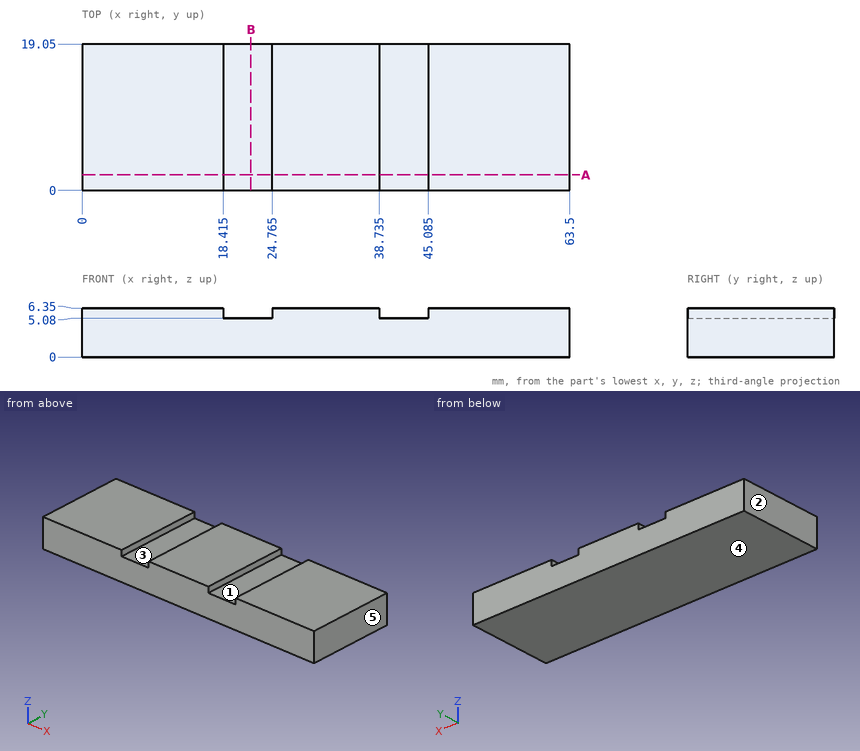
Job drawing, mm, ordinate dimensions from the low corner. One solid piece. A direction names the side the tool comes from. Coordinates: 2 decimals unless noted, no trailing zeros. Order: outer loops, then holes, each group sorted by start corner. A loop starts at its lowest first (then second) coordinate and runs counter-clockwise, first axis right, second up. Notation, with made-up numbers: (-28, -2.75) -> (27, -2.75) arc R28 ccw to (27, 21.25) -> close; hole circle Ø8 at (-27.5, 41.5). An arc over 180 degrees is marked (long way). Answer in a Markdown table with one row per item. Add a question column.
Q1. Wall check: line 1 along X through (y, z) = (8, 5.5) (3 decimals); line 2 along Z through (x, y) = (21, 1). Give the ranges that are in metal, low to high. Write a range as [from, to].
Q2. Band-saw the part on A-A, the plane y = 2. List the corners of the cut face in (x, z) (3 decimals).
Q3. Drop a flat-ended pin along its axis: pin 1 (1.9 mm diameter, centred on x = 23, y = 8.5, fed in from +Z). Give the stop position or say it passes through.
Q4. Band-saw the part on B-B, the plane x = 22. List the corners of the cut face in (y, z).
Q5. Mould opens along X. For the marked faces 3, 4 and 5 say: +X half, -X half, draft (parallel to the pull), parting line (faces both ways), or undercut.
Q6. Which spindle directions (+Z, -Z, +X, -X, +Y, -Y) get a long thin tool onto all of the face, cutting with end or side? Do the marked faces 1 and 2. Say none if no direction does.
Answers follow:
| question | item | result |
|---|---|---|
| 1 | line 1 | [0, 18.415], [24.765, 38.735], [45.085, 63.5] |
| 1 | line 2 | [0, 5.08] |
| 2 | outline | (0, 0) -> (63.5, 0) -> (63.5, 6.35) -> (45.085, 6.35) -> (45.085, 5.08) -> (38.735, 5.08) -> (38.735, 6.35) -> (24.765, 6.35) -> (24.765, 5.08) -> (18.415, 5.08) -> (18.415, 6.35) -> (0, 6.35) -> close |
| 3 | pin 1 | z = 5.08 |
| 4 | outline | (0, 0) -> (19.05, 0) -> (19.05, 5.08) -> (0, 5.08) -> close |
| 5 | face 3 | undercut |
| 5 | face 4 | draft |
| 5 | face 5 | +X half |
| 6 | face 1 | +Z, +Y, -Y |
| 6 | face 2 | +Z, -Z, -X, +Y, -Y |
